```python
from build123d import *

# Parameters (mm, degrees)
PAD_DEPTH    = 2.5
SKETCH001_R  = 3
PAD001_DEPTH = 5
SKETCH002_R  = 3.25
POCKET_DEPTH = 5


with BuildPart() as part:
    # Sketch → Pad (new body, symmetric)
    with BuildSketch(Plane.XY):
        with BuildLine():
            ThreePointArc((0, 90.5), (-63.993164, 63.993164), (-90.5, 0))
            Line((-100.5, 0), (-90.5, 0))
            ThreePointArc((0, 100.5), (-71.064232, 71.064232), (-100.5, 0))
            Line((0, 100.5), (0, 90.5))
        make_face()
    extrude(amount=PAD_DEPTH, both=True)

    # Sketch001 → Pad001 (new body)
    with BuildSketch(Plane.XY.offset(2.5)):
        with Locations((2, 95.5)):
            Circle(SKETCH001_R)
    extrude(amount=-PAD001_DEPTH)

    # Sketch002 → Pocket (cut)
    with BuildSketch(Plane.XY.offset(2.5)):
        with Locations((-95.5, 2)):
            Circle(SKETCH002_R)
    extrude(amount=-POCKET_DEPTH, mode=Mode.SUBTRACT)


solid = part.part
```
The listing builds one solid part. Answer for the finished solid, in the listing's coordinates (mm). Give positions to 0.01 mm unless a question says otherwise; leave off trailing zeros. Order: outer loops, then holes, each group sorted by start corner. A loop starts at its lowest first (then second) coordinate and runs counter-clockwise, first axis right, second up. Notation, with made-up numbers: (-3.75, 1.5) -> (21.25, 1.5) arc R13 cw to (21.25, 6.5) -> close; hole circle Ø9 at (76.25, 21.25). An arc over 180 degrees is marked (long way). Answer as a JSON object with one key per item and string values. Group by question number.
Item 1: The part is cut by section C-C on x = 2. Write down the section's boundary in (y, z).
Item 2: The part is cut by section D-D on y = 86. Write down the section's boundary in (x, z).
Item 3: Flat-ended cylindrical pins translate along their axes: pin 1 (8 mm diameter, centred on x = -78.5, y = 44, fed in from +Z); pin 2 (0.8 mm diameter, centred on y = 99.5, z = 0.5, fed in from +X); pin 3 (3 mm diameter, centred on x = -79.5, z = -1, fed in from +Y); pin 4 (1.5 mm diameter, centred on y = 76.5, z = 0, fed in from -X). Find the tip coordinate at first contact, or state that the pin passes through.
Item 4: The part is cut by section B-B on y = 2. Write down the section's boundary in (x, z), and give its area (3 significant figures).
Item 5: Consider L1, parallel to X at y = 2, z = -0.6; L2, parallel to X at y = 46.5, z = 0.9; L3, parallel to Y at x = -52.5, z = -0.6. Determine where each line is inside the solid, lowest interval first. Write a range as from..to.
Item 6: Determine the mould class of faces 1 (the cylindrical face through (5, 95.4, 0)), 2 (the cylindrical face through (-95.4, 5.25, 0.04)), 3 (the cylindrical face through (-70.28, 71.84, 0.04)), 4 (the flat face through (-64, 65, 2.5)) for opening direction X: pulls with the +X half, pulls with the -X half, needs draft (parallel to the pull), parting line crosses it, or undercut.
Item 7: The part is cut by section A-A on z = -0.65. Write down the section's boundary in (x, y), and give its area (3 significant figures).
Result set:
{
 "1": {"outline": "(92.5, -2.5) -> (98.5, -2.5) -> (98.5, 2.5) -> (92.5, 2.5) -> close"},
 "2": {"outline": "(-52, -2.5) -> (-28.18, -2.5) -> (-28.18, 2.5) -> (-52, 2.5) -> close"},
 "3": {"pin 1": "z = 2.5", "pin 2": "x = 0", "pin 3": "y = 63.37", "pin 4": "x = -66.05"},
 "4": {"outline": "(-100.48, -2.5) -> (-98.75, -2.5) -> (-98.75, 2.5) -> (-100.48, 2.5) -> close; (-92.25, -2.5) -> (-90.48, -2.5) -> (-90.48, 2.5) -> (-92.25, 2.5) -> close", "area": "17.5 mm²"},
 "5": {"L1": "-100.48..-98.75, -92.25..-90.48", "L2": "-89.1..-77.64", "L3": "73.72..85.7"},
 "6": {"face 1": "undercut", "face 2": "undercut", "face 3": "pulls with the -X half", "face 4": "needs draft"},
 "7": {"outline": "(-100.5, 0) -> (-98.06, 0) arc R3.25 cw (long way) to (-92.94, 0) -> (-90.5, 0) arc R90.5 cw to (0, 90.5) -> (0, 93.26) arc R3 ccw (long way) to (0, 97.74) -> (0, 100.5) arc R100.5 ccw to start", "area": "1,500 mm²"}
}
